Study the drawing (mm; zero at the part's minimum x, y, z) and answer. A direction names the side the tool comes from. Round coordinates to 2 decimals unless told otherwise and drop trailing zeros. Loops run counter-clockwise (first coordinate to the right, second up) from the corner with the lowest first, then second, coordinate; pieces in that order, holes last. Notation, with made-up numbers: (-1, -22) -> (24, -22) arc R35 cw to (24, 14) -> close; hole circle Ø9 at (8.5, -3). An arc over 180 degrees is marked (long way). Use one line per item in the form item = value.
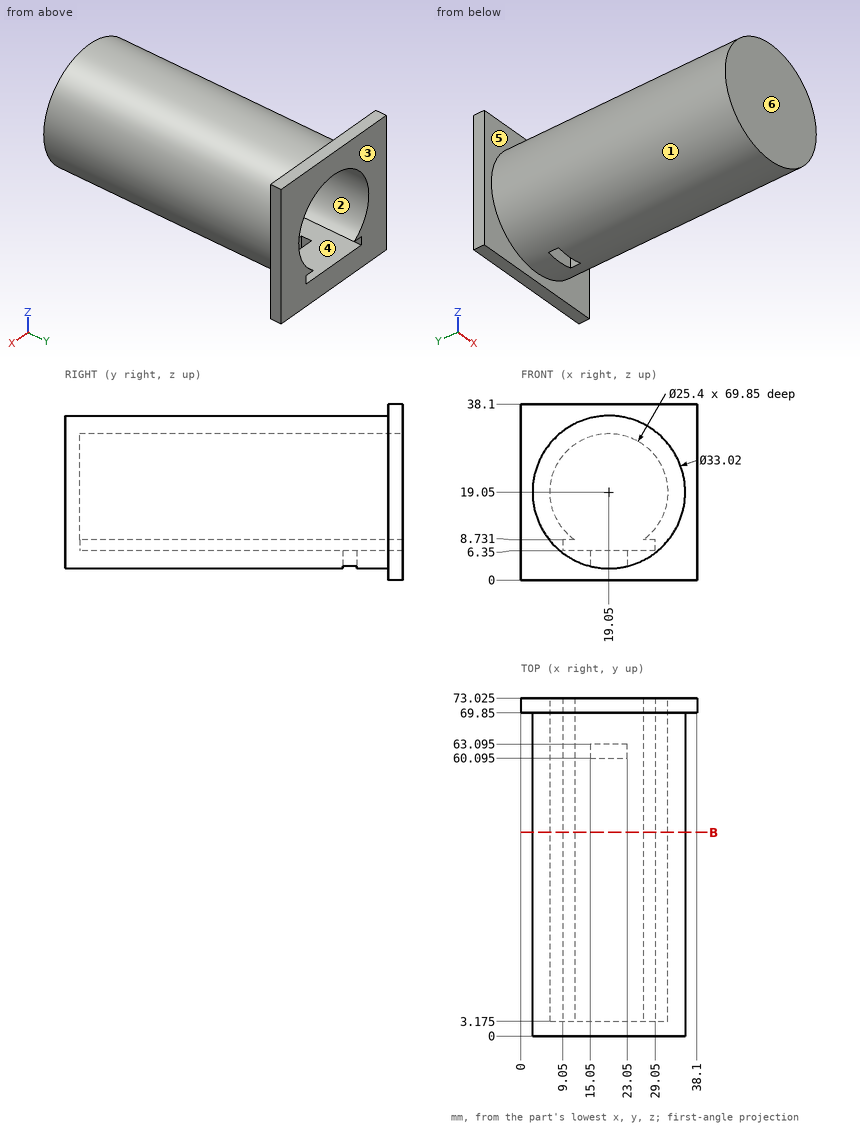
(1) Given P1, Ø3, axis at y = 42, z = 4.5, coming from the -X side; P2, Ø7.5, axis at x = 14, z = 23, coming from the +Y side (3 decimals); P3, Ø19, axis at x = 20.5, z = 16, coming from the -Y side; P4, Ø22, axis at x = 20.5, y = 30, coming from the +Z side, each flat-ended and moving along its own axis, determine where each tip first touches the part or whether it passes through.
Completed:
P1 = 8.94
P2 = 3.175
P3 = 0
P4 = 35.56
(2) Consider L1, parallel to X at y = 32, z = 19; L2, parallel to Y at x = 18.5, z = 3.5 (1 decimal). Determine where each line is inside the solid, lowest interval first.
Completed:
L1 = 2.54 to 6.35, 31.75 to 35.56
L2 = 0 to 60.1, 63.1 to 73
(3) For the marked faces 5 and 6, determine the directions among +Z, -Z, +X, -X, +Y, -Y from which every point of the face is accessible in a straight line to the end or side of a thin tool.
Completed:
face_5 = -Y
face_6 = +Z, -Z, +X, -X, -Y
(4) For a pull along X with two mould halves and no side action, classify the marked faces 1, 2, 3 and 4 as +X half, -X half, draft (parallel to the pull), parting line (faces both ways), or undercut.
Completed:
face_1 = parting line
face_2 = undercut
face_3 = draft
face_4 = undercut
(5) Find section B-B, the plane y = 44. Write down the section's boundary in (x, z).
Completed:
outline = circle Ø33.02 at (19.05, 19.05); hole (9.05, 6.35) -> (29.05, 6.35) -> (29.05, 8.73) -> (26.45, 8.73) arc R12.7 ccw (long way) to (11.65, 8.73) -> (9.05, 8.73) -> close
